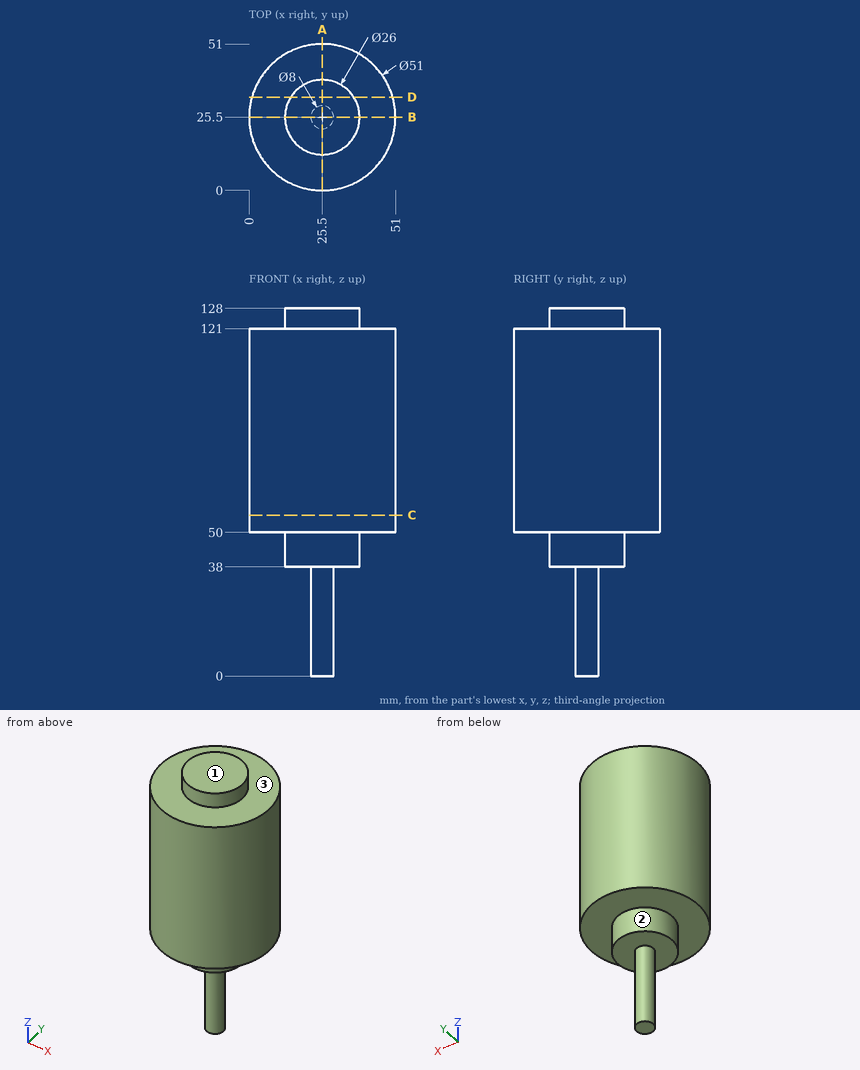
Can you work these out from the drawing? Everything is in mm from the part's minimum corner. A direction names the side the tool comes from. Coordinates: 2 decimals unless noted, no trailing zeros. Loops run counter-clockwise (first coordinate to the right, second up) from the corner with the lowest first, then second, coordinate; pieces in that order, holes last. Notation, with made-up numbers: (20, 69.5) - (32, 69.5) arc R35 ccw to (32, 108.5) - close; hole circle Ø8 at (13.25, 17). An arc over 180 degrees is marked (long way). Use a Markdown table: item, result.
Item 1: I want a section at A-A on x = 25.5. Please give me the cut outline in (y, z).
Numbers:
| item | result |
|---|---|
| outline | (0, 50) - (12.5, 50) - (12.5, 38) - (21.5, 38) - (21.5, 0) - (29.5, 0) - (29.5, 38) - (38.5, 38) - (38.5, 50) - (51, 50) - (51, 121) - (38.5, 121) - (38.5, 128) - (12.5, 128) - (12.5, 121) - (0, 121) - close |
Item 2: I want a section at C-C on z = 56. Please give me the cut outline in (x, y).
Numbers:
| item | result |
|---|---|
| outline | circle Ø51 at (25.5, 25.5) |
Item 3: For the marked faces 1, 2 and 3, which set-ups out of +Z, -Z, +X, -X, +Y, -Y let a thin tool reach every point of the face, with its end or its side?
Numbers:
| item | result |
|---|---|
| face 1 | +Z, +X, -X, +Y, -Y |
| face 2 | -Z |
| face 3 | +Z |
Item 4: I want a section at D-D on y = 32.5. Please give me the cut outline in (x, z).
Numbers:
| item | result |
|---|---|
| outline | (0.98, 50) - (14.55, 50) - (14.55, 38) - (36.45, 38) - (36.45, 50) - (50.02, 50) - (50.02, 121) - (36.45, 121) - (36.45, 128) - (14.55, 128) - (14.55, 121) - (0.98, 121) - close |
Item 5: Will these pins go through, and if not, where does the flat tip stop? pin 1 (6 mm diameter, centred on y = 30.5, z = 14.5, fed in from -X); pin 2 (8 mm diameter, centred on x = 11.5, y = 29.5, fed in from +Z); pin 3 (10 mm diameter, centred on x = 44, z = 70, fed in from +Y); pin 4 (4 mm diameter, centred on x = 18, y = 23, fed in from -Z).
Numbers:
| item | result |
|---|---|
| pin 1 | stops at x = 22.04 |
| pin 2 | stops at z = 128 |
| pin 3 | stops at y = 47.13 |
| pin 4 | stops at z = 38 |
Item 6: If I drill on probe 1 along Z at (x, y) = (23, 44); probe 2 along Z at (x, y) = (16.5, 32.5); probe 3 along X at (y, z) = (23, 30), over which ranges is the centre line in solid material (lowest first)? Write a range as from..to.
Numbers:
| item | result |
|---|---|
| probe 1 | z = 50..121 |
| probe 2 | z = 38..128 |
| probe 3 | x = 22.38..28.62 |
